from build123d import *

# Parameters (mm, degrees)
SKETCH1_W           = 30
SKETCH1_H           = 5
BOSS_EXTRUDE1_DEPTH = 80
SKETCH2_R           = 2
CUT_EXTRUDE1_DEPTH  = 10
SKETCH3_R           = 1
SKETCH3_R_2         = 4
CUT_EXTRUDE3_DEPTH  = 82.547532152
SKETCH5_W           = 30
SKETCH5_H           = 3
CUT_EXTRUDE4_DEPTH  = 2
SKETCH6_R           = 1
CUT_EXTRUDE5_DEPTH  = 82.449370777


with BuildPart() as part:
    # Sketch1 → Boss-Extrude1 (new body)
    with BuildSketch(Plane(origin=(0, 0, 0), x_dir=(1, 0, 0), z_dir=(0, 1, 0))):
        Rectangle(SKETCH1_W, SKETCH1_H)
    extrude(amount=BOSS_EXTRUDE1_DEPTH)

    # Sketch2 → Cut-Extrude1 (cut)
    with BuildSketch(Plane(origin=(0, 80, 0), x_dir=(1, 0, 0), z_dir=(0, 1, 0))):
        with Locations(Location((-5, 0, 0), (0, 0, 270))):
            Circle(SKETCH2_R)
        with Locations(Location((5, 0, 0), (0, 0, 270))):
            Circle(SKETCH2_R)
    extrude(amount=-CUT_EXTRUDE1_DEPTH, mode=Mode.SUBTRACT)

    # Sketch3 → Cut-Extrude3 (cut, through all)
    with BuildSketch(Plane.XY.offset(2.5)):
        with Locations((0, 23)):
            Circle(SKETCH3_R)
        with Locations((5.656854249, 20.656854249)):
            Circle(SKETCH3_R)
        with Locations((8, 15)):
            Circle(SKETCH3_R)
        with Locations((5.656854249, 9.343145751)):
            Circle(SKETCH3_R)
        with Locations((0, 7)):
            Circle(SKETCH3_R)
        with Locations((-5.656854249, 9.343145751)):
            Circle(SKETCH3_R)
        with Locations((-8, 15)):
            Circle(SKETCH3_R)
        with Locations((-5.656854249, 20.656854249)):
            Circle(SKETCH3_R)
        with Locations((0, 15)):
            Circle(SKETCH3_R_2)
    extrude(amount=-CUT_EXTRUDE3_DEPTH, mode=Mode.SUBTRACT)

    # Sketch5 → Cut-Extrude4 (cut)
    with BuildSketch(Plane.XY.offset(2.5)):
        with Locations((0, 37.5)):
            Rectangle(SKETCH5_W, SKETCH5_H)
    extrude(amount=-CUT_EXTRUDE4_DEPTH, mode=Mode.SUBTRACT)

    # Sketch6 → Cut-Extrude5 (cut, through all)
    with BuildSketch(Plane.XY.offset(0.5)):
        with Locations((0, 37.5)):
            Circle(SKETCH6_R)
    extrude(amount=-CUT_EXTRUDE5_DEPTH, mode=Mode.SUBTRACT)


solid = part.part
Verification items for the finished model (mm, model axes). A direction names the side the tool comes from. Coordinates: 2 decimals unless noted, no trailing zeros. Order: outer loops, then holes, each group sorted by start corner. A loop starts at its lowest first (then second) coordinate and runs counter-clockwise, first axis right, second up.
1. Scan lines: line 1 (Y direction, x = 0, z = -1.3); line 2 (Y direction, x = 0, z = 0.75); line 3 (X direction, y = 75.25, z = 0). Record each from-to range of solid material in increasing order.
Results found:
line 1: y = 0 to 6, 8 to 11, 19 to 22, 24 to 36.5, 38.5 to 80
line 2: y = 0 to 6, 8 to 11, 19 to 22, 24 to 36, 39 to 80
line 3: x = -15 to -7, -3 to 3, 7 to 15
2. Release check for a two-part mould opening along X. For faces 1 (the face through (0, 39, -2.5)), 2 (the face through (7, 75, 0)), 3 (the face through (15, 39, 0)) record: +X half, -X half, draft (parallel to the pull), parting line (faces both ways), or undercut.
Results found:
face 1: draft
face 2: undercut
face 3: +X half
3. Sectioned sample at A-A, the plane x = 8. Record the cut outline in (y, z).
Results found:
outline: (0, -2.5) - (14, -2.5) - (14, 2.5) - (0, 2.5) - close; (16, -2.5) - (80, -2.5) - (80, 2.5) - (39, 2.5) - (39, 0.5) - (36, 0.5) - (36, 2.5) - (16, 2.5) - close
4. Sectioned sample at D-D, the plane y = 15. Record the cut outline in (x, z).
Results found:
outline: (-15, -2.5) - (-9, -2.5) - (-9, 2.5) - (-15, 2.5) - close; (-7, -2.5) - (-4, -2.5) - (-4, 2.5) - (-7, 2.5) - close; (4, -2.5) - (7, -2.5) - (7, 2.5) - (4, 2.5) - close; (9, -2.5) - (15, -2.5) - (15, 2.5) - (9, 2.5) - close
5. Go/stop test with flat-tipped pins: pin 1 Ø2.5 at (x, y) = (5.66, 9.34) entering from +Z; pin 2 Ø5 at (x, y) = (0, 15) entering from -Z. Record where each tip stops, or that it passes through.
Results found:
pin 1: stops at z = 2.5
pin 2: passes through
6. Set-up check for faces 4 (the face through (-7, 75, 0)), 5 (the face through (-0.521, 18.966, 0.035)): record each of +Z, -Z, +X, -X, +Y, -Y from which the full face is reachable in a straight line by a thin tool's end or side.
Results found:
face 4: +Y
face 5: +Z, -Z
7. Sectioned sample at C-C, the plane x = 0. Record the cut outline in (y, z), and give its area (3 significant figures).
Results found:
outline: (0, -2.5) - (6, -2.5) - (6, 2.5) - (0, 2.5) - close; (8, -2.5) - (11, -2.5) - (11, 2.5) - (8, 2.5) - close; (19, -2.5) - (22, -2.5) - (22, 2.5) - (19, 2.5) - close; (24, -2.5) - (36.5, -2.5) - (36.5, 0.5) - (36, 0.5) - (36, 2.5) - (24, 2.5) - close; (38.5, -2.5) - (80, -2.5) - (80, 2.5) - (39, 2.5) - (39, 0.5) - (38.5, 0.5) - close
area: 328 mm2
8. Sectioned sample at B-B, the plane y = 23. Record the cut outline in (x, z), and give its area (3 significant figures).
Results found:
outline: (-15, -2.5) - (-1, -2.5) - (-1, 2.5) - (-15, 2.5) - close; (1, -2.5) - (15, -2.5) - (15, 2.5) - (1, 2.5) - close
area: 140 mm2
